Could you check a few things on this model? Use its own coordinates, in mm. A direction names the side the tool comes from. Round coordinates to 2 decimals unless told otherwise and drop trailing zeros. Loops run counter-clockwise (first coordinate to the right, second up) from the corner with the lowest first, then second, coordinate; pieces in that order, holes last. Notation, with made-up numbers: M -12.5,79 L -1.5,79 A19 cw -1.5,91 Z; hole C 11,73 d11. An arc over 180 degrees is marked long. Return JSON: item names as keys, results as strings. Group by question number.
```python
from build123d import *

# Parameters (mm, degrees)
SKETCH28_W                                   = 80
SKETCH28_H                                   = 80
BOSS_EXTRUDE1_DEPTH                          = 10
CBORE_FOR_M10_CHEESE_HEAD_SCREW1_D           = 12
CBORE_FOR_M10_CHEESE_HEAD_SCREW1_CBORE_D     = 25
CBORE_FOR_M10_CHEESE_HEAD_SCREW1_CBORE_DEPTH = 5
BOSS_EXTRUDE2_START                          = 5
SKETCH31_W                                   = 25
SKETCH31_H                                   = 24
SKETCH31_R                                   = 6
BOSS_EXTRUDE2_DEPTH                          = 5
SKETCH36_R                                   = 1
BOSS_EXTRUDE5_DEPTH                          = 5
SKETCH37_R                                   = 6.5
CUT_EXTRUDE1_DEPTH                           = 2.6
SKETCH38_R                                   = 1.1
CUT_EXTRUDE2_DEPTH                           = 64.398733217
SKETCH39_W                                   = 10.140014898
SKETCH39_H                                   = 20.185275771
SKETCH39_W_2                                 = 10.140014899
BOSS_EXTRUDE6_DEPTH                          = 18
CUT_EXTRUDE3_REACH                           = 73.95
SKETCH42_R                                   = 3
CUT_EXTRUDE4_DEPTH                           = 9
SKETCH43_R                                   = 1.011275837
CUT_EXTRUDE5_DEPTH                           = 67.446435697
CUT_EXTRUDE7_REACH                           = 72.05
SKETCH47_R                                   = 3
CUT_EXTRUDE8_DEPTH                           = 9
SKETCH48_R                                   = 1
CUT_EXTRUDE9_DEPTH                           = 65.394869849


with BuildPart() as part:
    # Sketch28 → Boss-Extrude1 (new body)
    with BuildSketch(Plane(origin=(0, 0, 0), x_dir=(1, 0, 0), z_dir=(0, 1, 0))):
        with Locations((1.944585414, 4.241283073)):
            Rectangle(SKETCH28_W, SKETCH28_H)
    extrude(amount=BOSS_EXTRUDE1_DEPTH)

    # CBORE for M10 Cheese Head Screw1 (through all)
    with Locations(Plane(origin=(0, 10, 0), x_dir=(1, 0, 0), z_dir=(0, 1, 0))):
        with Locations((1.944585414, 4.241283073)):
            CounterBoreHole(CBORE_FOR_M10_CHEESE_HEAD_SCREW1_D / 2, CBORE_FOR_M10_CHEESE_HEAD_SCREW1_CBORE_D / 2, CBORE_FOR_M10_CHEESE_HEAD_SCREW1_CBORE_DEPTH)

    # Sketch31 → Boss-Extrude2 (add)
    with BuildSketch(Plane(origin=(0, 0, 0), x_dir=(-1, 0, 0), z_dir=(0, -1, 0)).offset(BOSS_EXTRUDE2_START)):
        with Locations((-1.944585414, 6.741283073)):
            Rectangle(SKETCH31_W, SKETCH31_H)
        with Locations(Location((-1.944585414, 4.241283073, 0), (0, 0, 270))):
            Circle(SKETCH31_R, mode=Mode.SUBTRACT)
    extrude(amount=-BOSS_EXTRUDE2_DEPTH)

    # Sketch36 → Boss-Extrude5 (add)
    with BuildSketch(Plane.XZ.offset(5)):
        with Locations(Location((12.444585414, -16.741283073, 0), (0, 0, 90))):
            Circle(SKETCH36_R)
        with Locations(Location((12.444585414, -4.241283073, 0), (0, 0, 90))):
            Circle(SKETCH36_R)
        with Locations(Location((-8.555414586, -16.741283073, 0), (0, 0, 90))):
            Circle(SKETCH36_R)
        with Locations(Location((-8.555414586, -4.241283073, 0), (0, 0, 90))):
            Circle(SKETCH36_R)
    extrude(amount=BOSS_EXTRUDE5_DEPTH)

    # Sketch37 → Cut-Extrude1 (cut)
    with BuildSketch(Plane(origin=(0, 10, 0), x_dir=(1, 0, 0), z_dir=(0, 1, 0))):
        with Locations(Location((1.944585414, -15.067812269, 0), (0, 0, 270))):
            Circle(SKETCH37_R)
        with Locations(Location((1.944585414, 23.550378415, 0), (0, 0, 90))):
            Circle(SKETCH37_R)
    extrude(amount=-CUT_EXTRUDE1_DEPTH, mode=Mode.SUBTRACT)

    # Sketch38 → Cut-Extrude2 (cut, through all)
    with BuildSketch(Plane(origin=(0, 7.4, 0), x_dir=(1, 0, 0), z_dir=(0, 1, 0))):
        with Locations(Location((1.944585414, -19.467812269, 0), (0, 0, 270))):
            Circle(SKETCH38_R)
        with Locations(Location((-2.455414586, -15.067812269, 0), (0, 0, 270))):
            Circle(SKETCH38_R)
        with Locations(Location((1.944585414, -10.667812269, 0), (0, 0, 270))):
            Circle(SKETCH38_R)
        with Locations(Location((6.344585414, -15.067812269, 0), (0, 0, 270))):
            Circle(SKETCH38_R)
        with Locations(Location((1.944585414, 27.950378415, 0), (0, 0, 90))):
            Circle(SKETCH38_R)
        with Locations(Location((6.344585414, 23.550378415, 0), (0, 0, 90))):
            Circle(SKETCH38_R)
        with Locations(Location((1.944585414, 19.150378415, 0), (0, 0, 338.166857226))):
            Circle(SKETCH38_R)
        with Locations(Location((-2.455414586, 23.550378415, 0), (0, 0, 90))):
            Circle(SKETCH38_R)
    extrude(amount=-CUT_EXTRUDE2_DEPTH, mode=Mode.SUBTRACT)

    # Sketch39 → Boss-Extrude6 (add)
    with BuildSketch(Plane(origin=(-3.101061249, 10, 0), x_dir=(1, 0, 0), z_dir=(0, 1, 0))):
        with Locations((22.915466142, 2.76667369)):
            Rectangle(SKETCH39_W, SKETCH39_H)
        with Locations((-12.824172815, 2.76667369)):
            Rectangle(SKETCH39_W_2, SKETCH39_H)
    extrude(amount=BOSS_EXTRUDE6_DEPTH)

    # Sketch41 → Cut-Extrude3 (cut, up to next)
    with BuildSketch(Plane(origin=(-3.101061249, 0, -12.859311575), x_dir=(-1, 0, 0), z_dir=(0, 0, -1)), mode=Mode.PRIVATE) as cut_extrude3_sk1:
        Polygon((-17.845458693, 28), (-27.985473591, 28), (-17.845458693, 25.166138953), align=None)
    cut_extrude3_tool1 = extrude(cut_extrude3_sk1.sketch, amount=-CUT_EXTRUDE3_REACH, mode=Mode.PRIVATE) & part.part
    add(cut_extrude3_tool1.solids().sort_by_distance((18.124402, 27.05538, -12.859312))[0], mode=Mode.SUBTRACT)

    # Sketch42 → Cut-Extrude4 (cut)
    with BuildSketch(Plane(origin=(-8.331937614, 18.716924855, 0), x_dir=(0.9630956709984104, 0.2691592994940385, 0), z_dir=(-0.26915929949403855, 0.9630956709984105, 0))):
        with Locations(Location((29.519399999, 2.697534427, 0), (0, 0, 180))):
            Circle(SKETCH42_R)
    extrude(amount=-CUT_EXTRUDE4_DEPTH, mode=Mode.SUBTRACT)

    # Sketch43 → Cut-Extrude5 (cut, through all)
    with BuildSketch(Plane(origin=(-3.033104412, 10.852940003, 0), x_dir=(0.9630956709984104, 0.26915929949403844, 0), z_dir=(-0.2691592994940385, 0.9630956709984105, 0))):
        with Locations(Location((26.468109022, 1.00975317, 0), (0, 0, 180))):
            Circle(SKETCH43_R)
        with Locations(Location((26.468109022, 3.95432313, 0), (0, 0, 180))):
            Circle(SKETCH43_R)
    extrude(amount=-CUT_EXTRUDE5_DEPTH, mode=Mode.SUBTRACT)

    # Sketch46 → Cut-Extrude7 (cut, up to next)
    with BuildSketch(Plane(origin=(0, 0, -12.859311575), x_dir=(-1, 0, 0), z_dir=(0, 0, -1)), mode=Mode.PRIVATE) as cut_extrude7_sk1:
        Polygon((10.855226615, 25.166138953), (20.995241513, 28), (10.855226615, 28), align=None)
    cut_extrude7_tool1 = extrude(cut_extrude7_sk1.sketch, amount=-CUT_EXTRUDE7_REACH, mode=Mode.PRIVATE) & part.part
    add(cut_extrude7_tool1.solids().sort_by_distance((-14.235232, 27.05538, -12.859312))[0], mode=Mode.SUBTRACT)

    # Sketch47 → Cut-Extrude8 (cut)
    with BuildSketch(Plane(origin=(5.737295811, 20.528975847, 0), x_dir=(0.9630956709983024, -0.26915929949442535, 0), z_dir=(0.2691592994944253, 0.9630956709983023, 0))):
        with Locations(Location((-22.492604345, 2.766673689, 0), (0, 0, 180))):
            Circle(SKETCH47_R)
    extrude(amount=-CUT_EXTRUDE8_DEPTH, mode=Mode.SUBTRACT)

    # Sketch48 → Cut-Extrude9 (cut, through all)
    with BuildSketch(Plane(origin=(3.314862115, 11.861114808, 0), x_dir=(0.9630956709983024, -0.26915929949442546, 0), z_dir=(0.2691592994944254, 0.9630956709983023, 0))):
        with Locations(Location((-22.718123544, 4.075619229, 0), (0, 0, 180))):
            Circle(SKETCH48_R)
        with Locations(Location((-22.718123544, 1.383948503, 0), (0, 0, 180))):
            Circle(SKETCH48_R)
    extrude(amount=-CUT_EXTRUDE9_DEPTH, mode=Mode.SUBTRACT)


solid = part.part
```
1. We'd pull the mould along Z, two halves only. Please class faces 1 (the face through (2, -3, 5.259)), 2 (the face through (18.623, 21.643, -3.847)), 3 (the face through (-38.055, 5, -4)): +Z half, -Z half, draft (parallel to the pull), parting line (faces both ways), or undercut.
2. I need wall thicknesses on probe 1 along Z at (x, y) = (2, 7.5); probe 2 along Y at (x, z) = (24, -18); probe 3 along X at (y, z) = (5, -27.5). Which ranges of each line are inside material? Lowest first, please.
3. I'm going to push flat-ended pins straight in: pin 1 Ø9 at (y, z) = (21.5, -2.5) entering from +X; pin 2 Ø3.5 at (x, z) = (1.94, -27.95) entering from -Y; pin 3 Ø8 at (x, y) = (-15.5, 20.5) entering from +Z. Where does each tip first touch, or does it pass through?
4. If we section it at A-A, the plane x = 4: Please give me the cut outline in (y, z), then the cut area to 3 significant figures.
5. On a 3-axis mill with a long thin cutter (end or side, diameter ignored), from which of +Z, -Z, +X, -X, +Y, -Y can I reach the whole of each face in a straight line? I mean faces 4 (the face through (5, -5, -10)), 5 (the face through (24.884, 17, -3)), 6 (the face through (2, 7.4, -23)). Say none if no direction works.
6. If we section it at B-B, the plane y = 22: Give the number of separate pieces and of enclosed holes in the cut face, then the cut area to 3 significant figures.
7. If we section it at D-D, the plane x = -12: Please give me the cut outline in (y, z).
8. If we section it at C-C, the plane z = 26: Please give me the cut outline in (x, y).
Geometry results:
{
 "1": {"face 1": "+Z half", "face 2": "undercut", "face 3": "draft"},
 "2": {"probe 1": "-44.24 to -30.05, -17.05 to -16.74, 8.26 to 8.57, 21.57 to 35.76", "probe 2": "0 to 10", "probe 3": "-38.06 to 0.94, 2.95 to 41.94"},
 "3": {"pin 1": "x = 24.88", "pin 2": "y = 0", "pin 3": "z = 7.33"},
 "4": {"outline": "M -5,-18.74 L 0,-18.74 L 0,-44.24 L 10,-44.24 L 10,-29.72 L 7.4,-29.72 L 7.4,-17.38 L 10,-17.38 L 10,-16.57 L 5,-16.57 L 5,-9.88 L -5,-9.88 Z; M -5,1.4 L 5,1.4 L 5,8.09 L 10,8.09 L 10,8.9 L 7.4,8.9 L 7.4,21.23 L 10,21.23 L 10,35.76 L 0,35.76 L 0,5.26 L -5,5.26 Z", "area": "620 mm^2"},
 "5": {"face 4": "-Y", "face 5": "+Z, -Z, +X, +Y", "face 6": "+Y"},
 "6": {"separate pieces": "2", "enclosed holes": "2", "area": "351 mm^2"},
 "7": {"outline": "M 0,-44.24 L 10,-44.24 L 10,-12.86 L 25.49,-12.86 L 25.49,7.33 L 10,7.33 L 10,35.76 L 0,35.76 Z"},
 "8": {"outline": "M -38.06,0 L 41.94,0 L 41.94,10 L -38.06,10 Z"}
}
